Model file for the job. Use its own axes, mm. A direction names the side the tool comes from. Give positions to 0.01 mm unless a question says otherwise; leave off trailing zeros. Order: outer loops, then holes, each group sorted by start corner. A loop starts at its lowest first (then second) coordinate and runs counter-clockwise, first axis right, second up. Notation, with made-up numbers: (53, 68.25) - (85, 68.25) arc R36 cw to (85, 105.25) - close; hole circle Ø7 at (53, -22). An arc over 180 degrees is marked (long way). Use CSV: the item, a comma, the result in double quotes. Start each with the question number.
(1) Probe L1, parallel to Y at x = 63.5, z = 9; L2, parallel to X at y = -17, z = 17.5. List the from-to ranges inside material, lowest first.
(2) Band-saw the part on D-D, the plane z = 23.5. Give the cut face in (x, y), then the cut area to 3 significant figures.
(3) Tool access for faces 4 (the flat face through (-1, -63.5, 25)), 5 (the cylindrical face through (-64.88, -69.7, 19.72)): list every direction of +Z, -Z, +X, -X, +Y, -Y with a clear straight run to the whole face (end or side of a thin tool).
(4) Band-saw the part on C-C, the plane y = -61. Give the cut face in (x, z).
(5) Drop a flat-ended pin along its axis: pin 1 Ø6 at (x, y) = (15, 51.5) entering from +Z. Give the stop position or say it passes through.
(6) Band-saw the part on A-A, the plane z = 6. Give the cut face in (x, y).
(7) Band-saw the part on B-B, the plane x = -28.5. Give the cut face in (y, z), then the cut area to 3 significant figures.
(8) Pull direction X, two halves, no side cores. Call faces 1 (the flat face through (-1, 1, 0)), 2 (the cylindrical face through (62.12, -69.7, 19.72)), 3 (the cylindrical face through (-70.65, 70.49, 19.72)): +X half, -X half, draft (parallel to the pull), parting line (faces both ways), or undercut.
from build123d import *

# Parameters (mm, degrees)
SKETCH1_W           = 147
SKETCH1_H           = 147
SKETCH1_R           = 6.35
BOSS_EXTRUDE1_DEPTH = 10
SKETCH2_W           = 147
SKETCH2_H           = 147
SKETCH2_R           = 6.35
BOSS_EXTRUDE2_DEPTH = 30
FILLET1_R           = 10


with BuildPart() as part:
    # Sketch1 → Boss-Extrude1 (new body)
    with BuildSketch(Plane.XY):
        Rectangle(SKETCH1_W, SKETCH1_H)
        with Locations((-63.5, 63.5)):
            Circle(SKETCH1_R, mode=Mode.SUBTRACT)
        with Locations((63.5, 63.5)):
            Circle(SKETCH1_R, mode=Mode.SUBTRACT)
        with Locations((63.5, -63.5)):
            Circle(SKETCH1_R, mode=Mode.SUBTRACT)
        with Locations((-63.5, -63.5)):
            Circle(SKETCH1_R, mode=Mode.SUBTRACT)
    extrude(amount=BOSS_EXTRUDE1_DEPTH)

    # Sketch2 → Boss-Extrude2 (add)
    with BuildSketch(Plane.XY.offset(10)):
        Rectangle(SKETCH2_W, SKETCH2_H)
        with Locations((-63.5, -63.5)):
            Circle(SKETCH2_R, mode=Mode.SUBTRACT)
        with Locations((63.5, -63.5)):
            Circle(SKETCH2_R, mode=Mode.SUBTRACT)
        with Locations((63.5, 63.5)):
            Circle(SKETCH2_R, mode=Mode.SUBTRACT)
        with Locations((-63.5, 63.5)):
            Circle(SKETCH2_R, mode=Mode.SUBTRACT)
        with BuildLine():
            Line((-43.5, -63.5), (43.5, -63.5))
            ThreePointArc((43.5, -63.5), (57.642135624, -57.642135624), (63.5, -43.5))
            Line((63.5, -43.5), (63.5, 43.5))
            ThreePointArc((63.5, 43.5), (57.642135624, 57.642135624), (43.5, 63.5))
            Line((43.5, 63.5), (-43.5, 63.5))
            ThreePointArc((-43.5, 63.5), (-57.642135624, 57.642135624), (-63.5, 43.5))
            Line((-63.5, 43.5), (-63.5, -43.5))
            ThreePointArc((-63.5, -43.5), (-57.642135624, -57.642135624), (-43.5, -63.5))
        make_face(mode=Mode.SUBTRACT)
    extrude(amount=BOSS_EXTRUDE2_DEPTH)

    # Fillet1
    fillet1_edges = [part.edges().sort_by_distance(p)[0] for p in [
        (-73.5, -73.5, 20),
        (-73.5, 73.5, 20),
        (73.5, 73.5, 20),
        (73.5, -73.5, 20),
    ]]
    fillet(fillet1_edges, radius=FILLET1_R)


solid = part.part
Answer block:
1,L1,"y = -73.5 to -69.85, -57.15 to 57.15, 69.85 to 73.5"
1,L2,"x = -73.5 to -63.5, 63.5 to 73.5"
2,outline,"(-73.5, -63.5) arc R10 ccw to (-63.5, -73.5) - (63.5, -73.5) arc R10 ccw to (73.5, -63.5) - (73.5, 63.5) arc R10 ccw to (63.5, 73.5) - (-63.5, 73.5) arc R10 ccw to (-73.5, 63.5) - close; hole circle Ø12.7 at (-63.5, -63.5); hole circle Ø12.7 at (-63.5, 63.5); hole (-63.5, -43.5) arc R20 ccw to (-43.5, -63.5) - (43.5, -63.5) arc R20 ccw to (63.5, -43.5) - (63.5, 43.5) arc R20 ccw to (43.5, 63.5) - (-43.5, 63.5) arc R20 ccw to (-63.5, 43.5) - close; hole circle Ø12.7 at (63.5, -63.5); hole circle Ø12.7 at (63.5, 63.5)"
2,area,"5,230 mm2"
3,face 4,"+Z"
3,face 5,"+Z, -Z"
4,outline,"(-73.5, 0) - (-69.34, 0) - (-69.34, 40) - (-73.5, 40) - close; (-57.66, 0) - (57.66, 0) - (57.66, 40) - (53.18, 40) - (53.18, 10) - (-53.18, 10) - (-53.18, 40) - (-57.66, 40) - close; (69.34, 0) - (73.5, 0) - (73.5, 40) - (69.34, 40) - close"
5,pin 1,"stops at z = 10"
6,outline,"(-73.5, -63.5) arc R10 ccw to (-63.5, -73.5) - (63.5, -73.5) arc R10 ccw to (73.5, -63.5) - (73.5, 63.5) arc R10 ccw to (63.5, 73.5) - (-63.5, 73.5) arc R10 ccw to (-73.5, 63.5) - close; hole circle Ø12.7 at (-63.5, -63.5); hole circle Ø12.7 at (-63.5, 63.5); hole circle Ø12.7 at (63.5, -63.5); hole circle Ø12.7 at (63.5, 63.5)"
7,outline,"(-73.5, 0) - (73.5, 0) - (73.5, 40) - (63.5, 40) - (63.5, 10) - (-63.5, 10) - (-63.5, 40) - (-73.5, 40) - close"
7,area,"2,070 mm2"
8,face 1,"draft"
8,face 2,"undercut"
8,face 3,"-X half"
